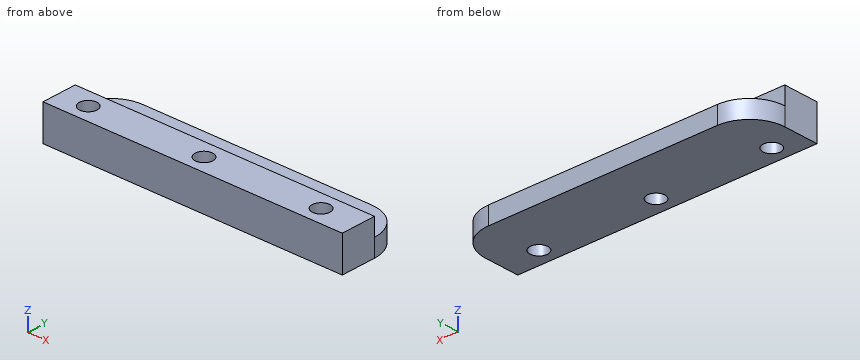
from build123d import *

# Parameters (mm, degrees)
F1_DEPTH = 6.35
F2_W     = 107.95
F2_H     = 12.7
F3_DEPTH = 6.35
F4_R     = 3.175
F5_DEPTH = 25.4


with BuildPart() as f1:
    # F0 (on Top) → F1 (new body)
    with BuildSketch(Plane.XY):
        with BuildLine():
            Line((0, 12.7), (0, 0))
            Line((0, 0), (107.95, 0))
            Line((107.95, 0), (107.95, 12.7))
            ThreePointArc((107.95, 12.7), (104.230256, 21.680256), (95.25, 25.4))
            Line((95.25, 25.4), (12.7, 25.4))
            ThreePointArc((12.7, 25.4), (3.719744, 21.680256), (0, 12.7))
        make_face()
    extrude(amount=F1_DEPTH)

    # F2 (on face) → F3 (join)
    with BuildSketch(Plane.XY.offset(6.35)):
        with Locations((53.975, 6.35)):
            Rectangle(F2_W, F2_H)
    extrude(amount=F3_DEPTH)

    # F4 (on face) → F5 (cut)
    with BuildSketch(Plane.XY.offset(12.7)):
        with Locations((10.503207, 6.35)):
            Circle(F4_R)
        with Locations((52.250076, 6.35)):
            Circle(F4_R)
        with Locations((94.490955, 6.35)):
            Circle(F4_R)
    extrude(amount=-F5_DEPTH, mode=Mode.SUBTRACT)


solid = f1.part
Geometry: final body of the model. Coordinates: model frame, mm. Give positions to 0.01 mm unless a question says otherwise; leave off trailing zeros. Loops run counter-clockwise (first coordinate to the right, second up) from the corner with the lowest first, then second, coordinate; pieces in that order, holes last. Notation, with made-up numbers: M 39.5,25 L 67.5,25 A5 ccw 67.5,32 Z; hole C 18.25,55 d9. An arc over 180 degrees is marked long. Put each result on its own line as item: value. Start each with the question number.
1) Contact query for flat-ended pins moving along their axis: pin 1 (1.9 mm diameter, centred on x = 72.5, z = 9, fed in from +Y); pin 2 (5 mm diameter, centred on x = 94.49, y = 6.35, fed in from -Z). Output: stop coordinate, or through.
2) Ray query, line 1 along Z through (x, y) = (59, 12.75); line 2 along Y through (x, z) = (75, 8). Return the intervals inside material, ascending.
3) Cut plane C-C (x = 60.5). Output: boundary loops of the cut face in (y, z), then the cut area to 3 significant figures.
4) Cut plane D-D (z = 2.5). Output: boundary loops of the cut face in (x, y) (3 decimals).
5) Cut plane B-B (z = 9.5). Output: boundary loops of the cut face in (x, y) (3 decimals), then the cut area to 3 significant figures.
6) Cut plane A-A (y = 6.35). Output: boundary loops of the cut face in (x, z), then the cut area to 3 significant figures.
Verdict:
1. pin 1: y = 12.7
1. pin 2: through
2. line 1: 0 to 6.35
2. line 2: 0 to 12.7
3. outline: M 0,0 L 25.4,0 L 25.4,6.35 L 12.7,6.35 L 12.7,12.7 L 0,12.7 Z
3. area: 242 mm2
4. outline: M 0,0 L 107.95,0 L 107.95,12.7 A12.7 ccw 95.25,25.4 L 12.7,25.4 A12.7 ccw 0,12.7 Z; hole C 10.503,6.35 d6.35; hole C 52.25,6.35 d6.35; hole C 94.491,6.35 d6.35
5. outline: M 0,0 L 107.95,0 L 107.95,12.7 L 0,12.7 Z; hole C 10.503,6.35 d6.35; hole C 52.25,6.35 d6.35; hole C 94.491,6.35 d6.35
5. area: 1,280 mm2
6. outline: M 0,0 L 7.33,0 L 7.33,12.7 L 0,12.7 Z; M 13.68,0 L 49.08,0 L 49.08,12.7 L 13.68,12.7 Z; M 55.43,0 L 91.32,0 L 91.32,12.7 L 55.43,12.7 Z; M 97.67,0 L 107.95,0 L 107.95,12.7 L 97.67,12.7 Z
6. area: 1,130 mm2
